from build123d import *

# Parameters (mm, degrees)
BOSS_EXTRUDE1_DEPTH = 5
SKETCH2_W           = 9.5
SKETCH2_H           = 5
BOSS_EXTRUDE2_DEPTH = 1
SKETCH3_R           = 2.5
BOSS_EXTRUDE3_DEPTH = 0.1


with BuildPart() as part:
    # Sketch1 → Boss-Extrude1 (new body)
    with BuildSketch(Plane.XY):
        Polygon((0, 0), (0, 5), (5, 1.498962309), (5, -10), (0, -10), align=None)
    extrude(amount=BOSS_EXTRUDE1_DEPTH)

    # Sketch2 → Boss-Extrude2 (add)
    with BuildSketch(Plane.XZ.offset(10)):
        with Locations((0.25, 2.5)):
            Rectangle(SKETCH2_W, SKETCH2_H)
    extrude(amount=BOSS_EXTRUDE2_DEPTH)

    # Sketch3 → Boss-Extrude3 (add)
    with BuildSketch(Plane.XZ.offset(11)):
        with Locations(Location((2.5, 2.5, 0), (0, 0, 270))):
            Circle(SKETCH3_R)
    extrude(amount=BOSS_EXTRUDE3_DEPTH)


solid = part.part
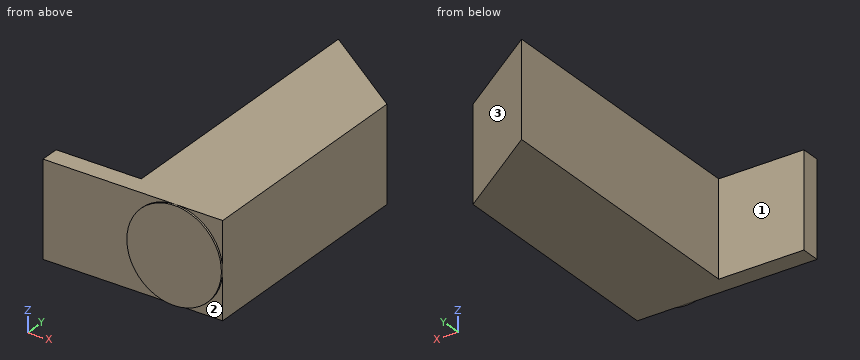
Verification items for the finished model (mm, model axes). Face numbers are marked on the shaded views. A direction names the side the tool comes from. Coordinates: 2 decimals unless noted, no trailing zeros. Order: outer loops, then holes, each group sorted by start corner. A loop starts at its lowest first (then second) coordinate and runs counter-clockwise, first axis right, second up.
1. Scan lines: line 1 (Y direction, x = -0.5, z = 3.6); line 2 (X direction, y = -1, z = 0.3); line 3 (X direction, y = 2.25, z = 1.6). Record each from-to range of solid material in increasing order.
Results found:
line 1: y = -11 to -10
line 2: x = 0 to 5
line 3: x = 0 to 3.93
2. Sectioned sample at C-C, the plane y = -5.25. Record the cut outline in (x, z).
Results found:
outline: (0, 0) - (5, 0) - (5, 5) - (0, 5) - close
3. Sectioned sample at D-D, the plane z = 3.95. Record the cut outline in (x, y).
Results found:
outline: (-4.5, -11) - (0.46, -11) - (0.46, -11.1) - (4.54, -11.1) - (4.54, -11) - (5, -11) - (5, 1.5) - (0, 5) - (0, -10) - (-4.5, -10) - close
4. Set-up check for the marked faces 1, 2 and 3: record each of +Z, -Z, +X, -X, +Y, -Y from which the full face is reachable in a straight line by a thin tool's end or side.
Results found:
face 1: +Z, -Z, -X, +Y
face 2: -Z, +X, -Y
face 3: +Z, -Z, +X, +Y
5. Go/stop test with flat-tipped pins: pin 1 Ø5 at (x, y) = (3, -7.5) entering from -Z; pin 2 Ø1.3 at (x, z) = (-1.5, 1.5) entering from +Y. Record where each tip stops, or that it passes through.
Results found:
pin 1: stops at z = 0
pin 2: stops at y = -10
6. Sectioned sample at B-B, the plane x = 1.25. Record the cut outline in (y, z), and give its area (3 significant figures).
Results found:
outline: (-11.1, 0.33) - (-11, 0.33) - (-11, 0) - (4.12, 0) - (4.12, 5) - (-11, 5) - (-11, 4.67) - (-11.1, 4.67) - close
area: 76.1 mm2
